Autodesk Inventor part; units mm, degrees
ref_plane "YZ Plane" through (0, 0, 0) normal (1, 0, 0) x (0, 1, 0)
ref_plane "XZ Plane" through (0, 0, 0) normal (0, 1, 0) x (-1, 0, 0)
sketch "スケッチ1" plane through (0, 0, 0) normal (0, 0, 1) x (1, 0, 0)
  line L0 (-3.1348, -0.9098) -> (10.2725, -0.9098) construction
  line L1 (10.2725, -0.9098) -> (10.2725, -4.9582) construction
  line L2 (10.2725, -4.9582) -> (-3.1348, -4.9582) construction
  line L3 (-3.1348, -4.9582) -> (-3.1348, -0.9098) construction
  line L4 (2.8417, -7.2866) -> (0.9879, -7.2866)
  line L5 (0.9879, -7.2866) -> (-0.6681, -4.8101)
  line L6 (-0.6681, -4.8101) -> (-0.9696, -5.2253)
  line L7 (-0.9696, -5.2253) -> (-0.9696, -7.2866)
  line L8 (-0.9696, -7.2866) -> (-2.502, -7.2866)
  line L9 (-2.502, -7.2866) -> (-2.502, -1.1866)
  line L10 (-2.502, -1.1866) -> (-0.9696, -1.1866)
  line L11 (-0.9696, -1.1866) -> (-0.9696, -3.9104)
  line L12 (-0.9696, -3.9104) -> (0.9879, -1.1866)
  line L13 (0.9879, -1.1866) -> (2.7527, -1.1866)
  line L14 (2.7527, -1.1866) -> (0.5776, -4.0191)
  line L15 (0.5776, -4.0191) -> (2.8417, -7.2866)
  spline S0 degree 2 poles (5.7928, -6.7973) (5.6445, -6.9208) (5.4122, -7.1186) (5.2144, -7.2174) knots 0 0 0 1 2 2 2
  spline S1 degree 2 poles (5.2144, -7.2174) (5.0216, -7.3114) (4.6558, -7.4102) (4.3296, -7.4102) knots 0 0 0 1 2 2 2
  spline S2 degree 2 poles (4.3296, -7.4102) (3.7166, -7.4102) (2.9109, -6.5896) (2.9109, -5.9668) knots 0 0 0 1 2 2 2
  spline S3 degree 2 poles (2.9109, -5.9668) (2.9109, -5.4576) (3.3212, -4.8249) (3.7067, -4.642) knots 0 0 0 1 2 2 2
  spline S4 degree 2 poles (3.7067, -4.642) (4.0973, -4.4542) (5.1798, -4.3059) (5.8027, -4.2663) knots 0 0 0 1 2 2 2
  line L16 (5.8027, -4.2663) -> (5.8027, -4.2416)
  spline S5 degree 2 poles (5.8027, -4.2416) (5.8027, -3.861) (5.2392, -3.5693) (4.6756, -3.5693) knots 0 0 0 1 2 2 2
  spline S6 degree 2 poles (4.6756, -3.5693) (4.4235, -3.5693) (3.7413, -3.7522) (3.42, -3.8956) knots 0 0 0 1 2 2 2
  line L17 (3.42, -3.8956) -> (3.2964, -3.8956)
  line L18 (3.2964, -3.8956) -> (3.2964, -2.7833)
  spline S7 degree 2 poles (3.2964, -2.7833) (3.509, -2.724) (4.4581, -2.5559) (4.9426, -2.5559) knots 0 0 0 1 2 2 2
  spline S8 degree 2 poles (4.9426, -2.5559) (6.1289, -2.5559) (7.2165, -3.3469) (7.2165, -4.1576) knots 0 0 0 1 2 2 2
  line L19 (7.2165, -4.1576) -> (7.2165, -7.2866)
  line L20 (7.2165, -7.2866) -> (5.7928, -7.2866)
  line L21 (5.7928, -7.2866) -> (5.7928, -6.7973)
  line L22 (5.7928, -6.0854) -> (5.7928, -5.1314)
  spline S9 degree 2 poles (5.7928, -5.1314) (5.427, -5.166) (4.9772, -5.2204) (4.7597, -5.2995) knots 0 0 0 1 2 2 2
  spline S10 degree 2 poles (4.7597, -5.2995) (4.5669, -5.3637) (4.3593, -5.6307) (4.3593, -5.8482) knots 0 0 0 1 2 2 2
  spline S11 degree 2 poles (4.3593, -5.8482) (4.3593, -6.1695) (4.7102, -6.4117) (5.0513, -6.4117) knots 0 0 0 1 2 2 2
  spline S12 degree 2 poles (5.0513, -6.4117) (5.2392, -6.4117) (5.6346, -6.2387) (5.7928, -6.0854) knots 0 0 0 1 2 2 2
  spline S13 degree 2 poles (10.2269, -7.3657) (10.2269, -8.1468) (9.3025, -9.0168) (8.5709, -9.0168) knots 0 0 0 1 2 2 2
  spline S14 degree 2 poles (8.5709, -9.0168) (8.1755, -9.0168) (7.5378, -8.9476) (7.3895, -8.908) knots 0 0 0 1 2 2 2
  line L23 (7.3895, -8.908) -> (7.3895, -7.8502)
  line L24 (7.3895, -7.8502) -> (7.4982, -7.8502)
  spline S15 degree 2 poles (7.4982, -7.8502) (7.6416, -7.8947) (7.9777, -7.949) (8.0815, -7.949) knots 0 0 0 1 2 2 2
  spline S16 degree 2 poles (8.0815, -7.949) (8.4968, -7.949) (8.7934, -7.4399) (8.7934, -6.8615) knots 0 0 0 1 2 2 2
  line L25 (8.7934, -6.8615) -> (8.7934, -3.683)
  line L26 (8.7934, -3.683) -> (7.9678, -3.683)
  line L27 (7.9678, -3.683) -> (7.9678, -2.6845)
  line L28 (7.9678, -2.6845) -> (10.2269, -2.6845)
  line L29 (10.2269, -2.6845) -> (10.2269, -7.3657)
  line L30 (10.2269, -2.027) -> (8.6994, -2.027)
  line L31 (8.6994, -2.027) -> (8.6994, -0.9098)
  line L32 (8.6994, -0.9098) -> (10.2269, -0.9098)
  line L33 (10.2269, -0.9098) -> (10.2269, -2.027)
  line L34 (12.7579, -7.2866) -> (11.3243, -7.2866)
  line L35 (11.3243, -7.2866) -> (11.3243, -2.6845)
  line L36 (11.3243, -2.6845) -> (12.7579, -2.6845)
  line L37 (12.7579, -2.6845) -> (12.7579, -7.2866)
  line L38 (12.8024, -2.027) -> (11.2848, -2.027)
  line L39 (11.2848, -2.027) -> (11.2848, -0.9098)
  line L40 (11.2848, -0.9098) -> (12.8024, -0.9098)
  line L41 (12.8024, -0.9098) -> (12.8024, -2.027)
  point P0 (0, 0)
extrude "押し出し1" add sketch "スケッチ1" along normal blind 0.3
ref_plane "作業平面1" through (0, 0, 0.3) normal (0, 0, 1) x (1, 0, 0)
sketch "スケッチ4" plane through (0, 0, 0.3) normal (0, 0, 1) x (1, 0, 0)
  line L0 (12.7579, -7.2866) -> (12.7579, -2.6845)
  line L1 (-2.502, -1.1866) -> (-2.502, -7.2866)
  line L2 (1.5924, -6.8642) -> (3.6217, -6.8642)
  line L3 (3.6217, -6.8642) -> (3.6217, -5.7481)
  line L4 (3.6217, -5.7481) -> (1.5924, -5.7481)
  line L5 (1.5924, -5.7481) -> (1.5924, -6.8642)
  line L6 (7.2165, -7.2866) -> (7.2165, -4.1576)
  line L7 (7.2165, -6.3062) -> (8.8066, -6.3062)
  line L8 (8.8066, -6.3062) -> (8.8066, -5.3089)
  line L9 (8.8066, -5.3089) -> (7.2165, -5.3089)
  line L10 (7.2165, -5.3089) -> (7.2165, -6.3062)
  line L11 (11.3243, -2.6845) -> (11.3243, -7.2866)
  line L12 (10.1491, -6.3062) -> (11.3243, -6.3062)
  line L13 (11.3243, -6.3062) -> (11.3243, -5.234)
  line L14 (11.3243, -5.234) -> (10.1491, -5.234)
  line L15 (10.1491, -5.234) -> (10.1491, -6.3062)
  line L16 (9.1301, -2.6845) -> (9.6378, -2.6845)
  line L17 (9.6378, -2.6845) -> (9.6378, -1.9909)
  line L18 (9.6378, -1.9909) -> (9.1301, -1.9909)
  line L19 (9.1301, -1.9909) -> (9.1301, -2.6845)
  line L20 (11.8767, -2.8267) -> (12.226, -2.8267)
  line L21 (12.226, -2.8267) -> (12.226, -1.8839)
  line L22 (12.226, -1.8839) -> (11.8767, -1.8839)
  line L23 (11.8767, -1.8839) -> (11.8767, -2.8267)
  point P0 (0, 0)
  dimension "d6" = 15.2599
extrude "押し出し3" add sketch "スケッチ4" against normal blind 0.3 contours L5 L4 L3 L2 | L6 L9 L8 L7 | L11 L12 L15 L14
extrude "押し出し4" add sketch "スケッチ4" against normal blind 0.3 contours L19 L18 L17 L16 | L23 L22 L21 L20
properties part number "photon_sample"
Here's how the part is built. I have some questions about the finished solid (model axes, mm). Round coordinates to 2 decimals unless told otherwise and drop trailing zeros. Write each loop counter-clockwise with the first axis right and the second up, starting at its lowest first coordinate (ties: lowest second). Pieces come first, ordered by that corner, then holes.
Q1. If we section it at B-B on x = -0.5: Write out the boundary of the cut face in (y, z).
Q2. If we section it at A-A on x = 11: Write out the boundary of the cut face in (y, z).
Q3. Please list where these lines run through material, in increasing order: probe 1 along X at (y, z) = (-3, 0.1); probe 2 along X at (y, z) = (-2.5, 0.15); probe 3 along X at (y, z) = (-6.75, 0.2).
Answer below:
1. outline: (-5.06, 0) - (-3.26, 0) - (-3.26, 0.3) - (-5.06, 0.3) - close
2. outline: (-6.31, 0) - (-5.23, 0) - (-5.23, 0.3) - (-6.31, 0.3) - close
3. probe 1: x = -2.5 to -0.97, -0.32 to 1.36, 3.3 to 6.74, 7.97 to 10.23, 11.32 to 12.76
3. probe 2: x = -2.5 to -0.97, 0.04 to 1.74, 9.13 to 9.64, 11.88 to 12.23
3. probe 3: x = -2.5 to -0.97, 0.63 to 7.22, 8.79 to 10.23, 11.32 to 12.76
